Can you work these out from the model? Positions are in its coordinate system, mm. Give positions to 0.01 mm unless a question says otherwise; leave off trailing zeros. Loops run counter-clockwise (first coordinate to the right, second up) from the corner with the lowest first, then second, coordinate; pieces in that order, holes last. Notation, with made-up numbers: (54, 71) -> (58, 71) arc R18 cw to (58, 87) -> close; hole circle Ø11 at (81, 62.5). An arc over 180 degrees is marked (long way). Return JSON: item names as keys, results as strings. Group by question number.
Q1. Will this pin go through, and if not, where does the flat tip stop? pin 1 (2 mm diameter, centred on y = 6, z = -13.5, fed in from -X).
Q2. Suppose I cut it at C-C, the plane z = -19.5. Please give me the cut outline in (x, y), and give its area (3 significant figures).
Q3. Thinking about a two-plate mould opening in X: for faces 1 (the cylindrical face through (15.738, -4.956, 0.651)), 2 (the cylindrical face through (6.691, 12.864, -0.735)), 3 (the flat face through (16, -1, 52.5)), which applies, pulls with the +X half, pulls with the -X half, needs draft (parallel to the pull), parting line crosses it, or undercut?
Q4. I need wall thicknesses on line 1 along Z through (x, y) = (39.5, 9); line 2 along Y through (x, z) = (0, 2); line 3 along Y through (x, z) = (12, 23). Which ranges of each line are inside material? Lowest first, please. Write a range as [from, to].
```python
from build123d import *

# Parameters (mm, degrees)
FILLET1_R = 3


with BuildPart() as part:
    # Sketch1 → Revolve1 (revolve)
    with BuildSketch(Plane(origin=(0, 0, 0), x_dir=(0, 0, -1), z_dir=(1, 0, 0)), mode=Mode.PRIVATE) as revolve1_sk:
        Polygon((-52.5, 80), (-52.5, 14.5), (52.5, 14.5), (52.5, 80), (46.5, 80), (46.5, 16.5), (-46.5, 16.5), (-46.5, 80), align=None)
    revolve(revolve1_sk.sketch.rotate(Axis((0, 0, 0), (0, 0, -1)), 90), axis=Axis((0, 0, 0), (0, 0, -1)))

    # Fillet1
    fillet1_edges = [part.edges().sort_by_distance(p)[0] for p in [
        (-80, 0, 46.5),
        (-80, 0, -46.5),
        (-80, 0, -52.5),
        (-80, 0, 52.5),
    ]]
    fillet(fillet1_edges, radius=FILLET1_R - 0.0001)  # a hair under: the kernel refuses the full size


solid = part.part
```
Ans:
{
 "1": {"pin 1": "stops at x = -15.72"},
 "2": {"outline": "circle Ø33 at (0, 0); hole circle Ø29 at (0, 0)", "area": "195 mm^2"},
 "3": {"face 1": "parting line crosses it", "face 2": "undercut", "face 3": "needs draft"},
 "4": {"line 1": "z = [-52.5, -46.5], [46.5, 52.5]", "line 2": "y = [-16.5, -14.5], [14.5, 16.5]", "line 3": "y = [-11.32, -8.14], [8.14, 11.32]"}
}
